from build123d import *

# Parameters (mm, degrees)
F0_W     = 38.1
F0_H     = 88.9
F1_DEPTH = 495.3
F2_SIZE2 = 88.89999
F2_SIZE  = 88.89999
F3_SIZE2 = 88.89999
F3_SIZE  = 88.89999


# Not quite as in the source:
# - a fillet or chamfer is up to 0.001 mm smaller than in the source, because OpenCascade refuses the exact size


with BuildPart() as f1:
    # F0 (on Front) → F1 (new body, symmetric)
    with BuildSketch(Plane.XZ):
        Rectangle(F0_W, F0_H)
    extrude(amount=F1_DEPTH, both=True)

    # F2 (size 88.9 and 88.9 in the source; OpenCascade refuses exactly that, so slightly less here)
    f2_edges = [f1.edges().sort_by_distance(p)[0] for p in [
        (0, -495.3, -44.45),
    ]]
    chamfer(f2_edges, length=F2_SIZE, length2=F2_SIZE2)

    # F3 (size 88.9 and 88.9 in the source; OpenCascade refuses exactly that, so slightly less here)
    f3_edges = [f1.edges().sort_by_distance(p)[0] for p in [
        (0, 495.3, -44.45),
    ]]
    chamfer(f3_edges, length=F3_SIZE, length2=F3_SIZE2)


solid = f1.part
Design review of the part built by this model. Coordinates are the model's own, in mm. Coordinates: 2 decimals unless noted, no trailing zeros. Order: outer loops, then holes, each group sorted by start corner. A loop starts at its lowest first (then second) coordinate and runs counter-clockwise, first axis right, second up. Notation, with made-up numbers: M 31,48.25 L 43,48.25 A10 cw 43,64.25 Z; hole C 67,-3.5 d3. An arc over 180 degrees is marked long. Use a Markdown table: item, result.
(1) For P1, Ø1.5, axis at x = 6, z = 27, coming from the +Y side; P2, Ø3, axis at x = 13, z = -13, coming from the +Y side, all flat-tipped, find the tip position at first contact; note any pin that passes through.
Worked answers:
| item | result |
|---|---|
| P1 | stops at y = 478.6 |
| P2 | stops at y = 439.35 |
(2) Wall thickness on probe 1 along Y at (x, z) = (-17, 13.5); probe 2 along Y at (x, z) = (-12, -7.5); probe 3 along Z at (x, y) = (-16, 453): over which ranges is each line inside the solid? List them lowest first.
Worked answers:
| item | result |
|---|---|
| probe 1 | y = -464.35 to 464.35 |
| probe 2 | y = -443.35 to 443.35 |
| probe 3 | z = 2.15 to 44.45 |
(3) Add section C-C (z = -24). Give the boundary of the cut face in (x, y), then the cut area to 3 significant figures.
Worked answers:
| item | result |
|---|---|
| outline | M -19.05,-426.85 L 19.05,-426.85 L 19.05,426.85 L -19.05,426.85 Z |
| area | 32,500 mm2 |
(4) Add section B-B (z = 19). Give the boundary of the cut face in (x, y).
Worked answers:
| item | result |
|---|---|
| outline | M -19.05,-469.85 L 19.05,-469.85 L 19.05,469.85 L -19.05,469.85 Z |
